Check sheet for the drawn part. Datum: minimum x, y, z corner. Units: mm. A direction names the side the tool comes from. Give positions to 0.01 mm unless a question says otherwise; leave off trailing zeros. Write each loop counter-clockwise with the first axis right and the second up, starting at its lowest first coordinate (ties: lowest second). Pieces come first, ordered by that corner, then holes. Notation, with made-up numbers: (85, 81.5) -> (95, 81.5) arc R10 ccw to (95, 94.5) -> close; hole circle Ø4 at (61, 7.25). An arc over 180 degrees is marked (long way). Write item = value, one per line. Start each with the question number.
1. Cross-section at C-C, the plane z = 24. State how many separate pieces and enclosed holes the cut face has, plus the area to 3 significant figures.
2. Cross-section at B-B, the plane x = 8. Record the cut outline in (y, z), plus the area to 3 significant figures.
3. Thickness scan on line 1 along X through (y, z) = (0.6, 45.92); line 2 along Z through (x, y) = (27, 2.6); line 3 along Z through (x, y) = (24.5, 1.9). Record the ranges inside material, lowest first.
4. Depth check by flat-ended pin: P1, Ø1, axis at y = 1.5, z = 14.5, coming from the +X side; P2, Ø0.9, axis at y = 1, z = 42.5, coming from the -X side; P3, Ø4.5, axis at x = 24.895, z = 3.87, coming from the +Y side. Enter the tip coordinate at first touch or a pass-through.
5. Cross-section at A-A, the plane y = 2.3. Record the cut outline in (x, z) (3 decimals).
6. Set-up check for the marked faces 1, 2, 3, 4 and 5: record each of +Z, -Z, +X, -X, +Y, -Y from which the full face is reachable in a straight line by a thin tool's end or side.
7. Cross-section at D-D, the plane z = 11.5. Record the cut outline in (x, y), plus the area to 3 significant figures.
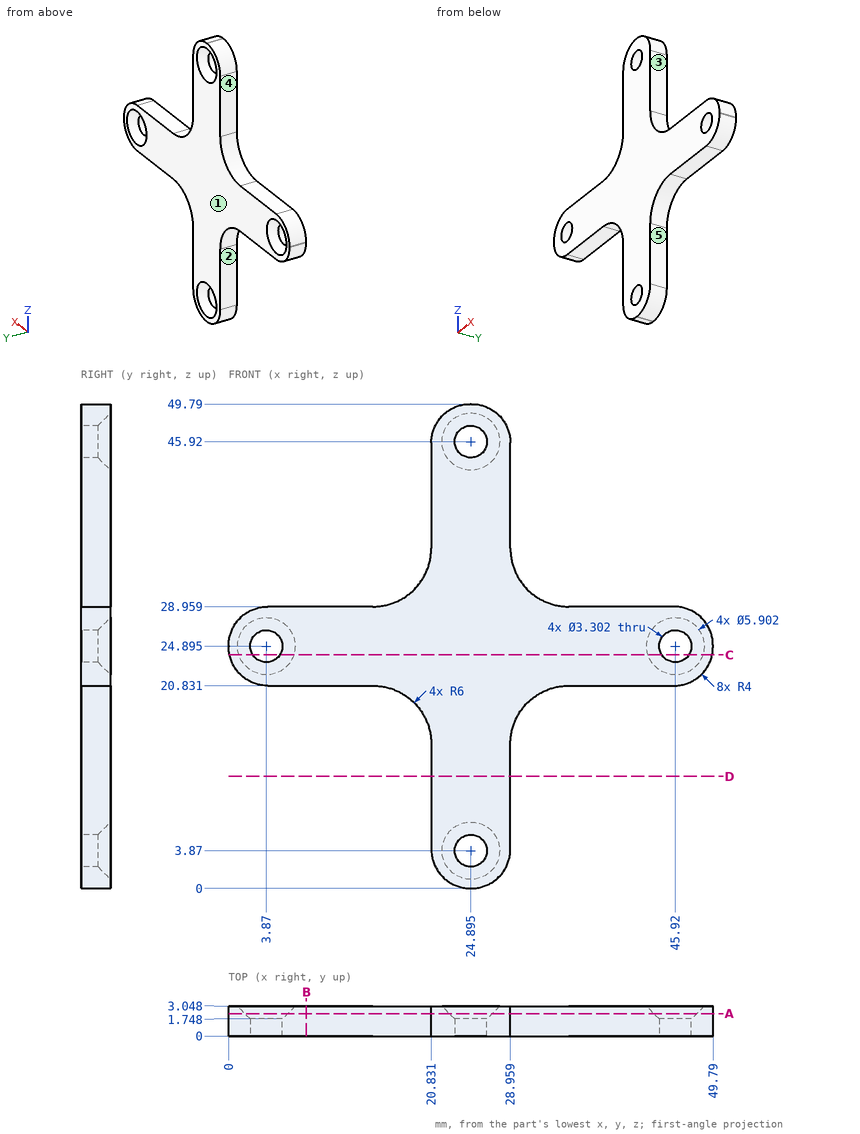
Answers:
q1.separate_pieces = 3
q1.enclosed_holes = 0
q1.area = 131 mm^2
q2.outline = (0, 20.83) -> (3.05, 20.83) -> (3.05, 28.96) -> (0, 28.96) -> close
q2.area = 24.8 mm^2
q3.line_1 = 20.83 to 23.24, 26.55 to 28.96
q3.line_2 = 0.56 to 2.52, 5.22 to 44.57, 47.27 to 49.23
q3.line_3 = 0.01 to 2.11, 5.63 to 44.16, 47.68 to 49.78
q4.P1 = 28.96
q4.P2 = 20.83
q4.P3 = 2.35
q5.outline = (0, 24.831) arc R4 ccw to (4, 20.831) -> (14.831, 20.831) arc R6 cw to (20.831, 14.831) -> (20.831, 4) arc R4 ccw to (24.831, 0) -> (24.959, 0) arc R4 ccw to (28.959, 4) -> (28.959, 14.831) arc R6 cw to (34.959, 20.831) -> (45.79, 20.831) arc R4 ccw to (49.79, 24.831) -> (49.79, 24.959) arc R4 ccw to (45.79, 28.959) -> (34.959, 28.959) arc R6 cw to (28.959, 34.959) -> (28.959, 45.79) arc R4 ccw to (24.959, 49.79) -> (24.831, 49.79) arc R4 ccw to (20.831, 45.79) -> (20.831, 34.959) arc R6 cw to (14.831, 28.959) -> (4, 28.959) arc R4 ccw to (0, 24.959) -> close; hole circle Ø4.406 at (3.87, 24.895); hole circle Ø4.406 at (24.895, 3.87); hole circle Ø4.406 at (24.895, 45.92); hole circle Ø4.406 at (45.92, 24.895)
q6.face_1 = +Z, -Z, +X, -X, +Y
q6.face_2 = -Z, -X, +Y, -Y
q6.face_3 = +Z, +X, +Y, -Y
q6.face_4 = +Z, -X, +Y, -Y
q6.face_5 = -Z, +X, +Y, -Y
q7.outline = (20.83, 0) -> (28.96, 0) -> (28.96, 3.05) -> (20.83, 3.05) -> close
q7.area = 24.8 mm^2
